Design review of the part built by this model. Coordinates are the model's own, in mm. Face numbers are marked on the shaded views. A direction names the side the tool comes from. Give positions to 0.01 mm unless a question says otherwise; leave off trailing zeros. Write each loop counter-clockwise with the first axis right and the second up, starting at its lowest first coordinate (ties: lowest second). Pieces come first, ordered by that corner, then holes.
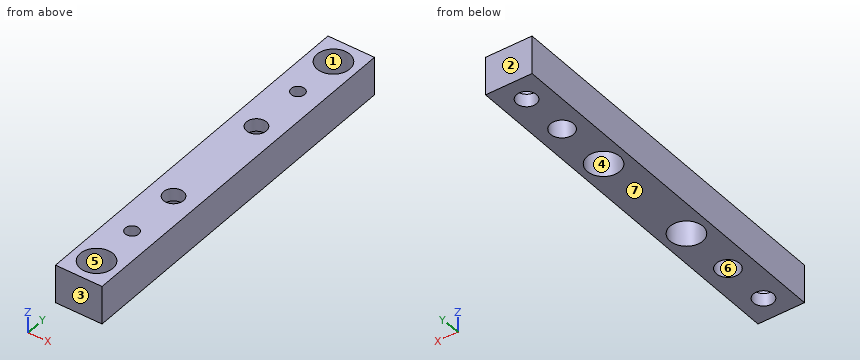
Solid Edge part; units mm, degrees
sketch "Sketch1" plane through (0, 0, 0) normal (0, 0, 1) x (1, 0, 0)
  line L0 (-7.25, -57.5) -> (7.25, -57.5)
  line L1 (7.25, -57.5) -> (7.25, 57.5)
  line L2 (7.25, 57.5) -> (-7.25, 57.5)
  line L3 (-7.25, 57.5) -> (-7.25, -57.5)
  dimension "D1" = 7.25
  dimension "D2" = 7.25
extrude "Protrusion1" add sketch "Sketch1" along normal blind 12
sketch "Sketch2" plane through (0, 0, 0) normal (0, 0, -1) x (0, -1, 0)
  circle A0 centre (-35, 0) radius 2.1
  circle A1 centre (-50, 0) radius 3.1
  circle A2 centre (-17.5, 0) radius 3.1
  dimension "D1" = 0
  dimension "D2" = 0
extrude "Cutout1" cut sketch "Sketch2" against normal up to next
sketch "Sketch3" plane through (0, 0, 0) normal (0, 0, -1) x (0, -1, 0)
  circle A0 centre (-17.5, 0) radius 5.1
  circle A1 centre (-35, 0) radius 3.6
extrude "ExtrudedCutout_2" cut sketch "Sketch3" against normal blind 8
sketch "Sketch4" plane through (0, 0, 12) normal (0, 0, 1) x (0, -1, 0)
  circle A0 centre (-50, 0) radius 5.1
extrude "ExtrudedCutout_3" cut sketch "Sketch4" against normal blind 8
mirror "Mirror1" about plane through (0, 0, 0) normal (0, 1, 0) of "Cutout1", "ExtrudedCutout_2", "ExtrudedCutout_3"
(1) To check wall thickness, follow L1, parallel to Y at x = 4, z = 10; L2, parallel to X at y = 35, z = 4; L3, parallel to Y at x = 3.75, z = 10.75. State the ranges of each line that lie inside material, in increasing order.
Resolved:
L1: y = -57.5 to -53.16, -46.84 to 46.84, 53.16 to 57.5
L2: x = -7.25 to -3.6, 3.6 to 7.25
L3: y = -57.5 to -53.46, -46.54 to 46.54, 53.46 to 57.5
(2) Consider section B-B, the plane y = -35. Give the boundary of the cut face in (x, z).
Resolved:
outline: (-7.25, 0) - (-3.6, 0) - (-3.6, 8) - (-2.1, 8) - (-2.1, 12) - (-7.25, 12) - close; (2.1, 8) - (3.6, 8) - (3.6, 0) - (7.25, 0) - (7.25, 12) - (2.1, 12) - close
(3) Mouldability with a two-part tool opening along Y and no side actions: class the marked faces 1, 2, 3 and 4 as pulls with the +Y half, pulls with the -Y half, needs draft (parallel to the pull), parting line crosses it, or undercut.
Resolved:
face 1: undercut
face 2: pulls with the +Y half
face 3: pulls with the -Y half
face 4: undercut
(4) Tool access review of the marked faces 5, 6 and 7: name each direction out of +Z, -Z, +X, -X, +Y, -Y from which nothing blocks a thin tool from reaching the whole face with its end or side.
Resolved:
face 5: +Z
face 6: -Z
face 7: -Z, +X, -X, +Y, -Y
(5) Consider section A-A, the plane z = 5.75. Give the boundary of the cut face in (x, y), then the cut area to 3 significant figures.
Resolved:
outline: (-7.25, -57.5) - (7.25, -57.5) - (7.25, 57.5) - (-7.25, 57.5) - close; hole circle Ø10.2 at (0, -50); hole circle Ø10.2 at (0, -17.5); hole circle Ø10.2 at (0, 17.5); hole circle Ø10.2 at (0, 50); hole circle Ø7.2 at (0, -35); hole circle Ø7.2 at (0, 35)
area: 1,260 mm2
(6) Clearance check with flat-ended pins moving along their axes: P1, Ø5, axis at x = -0.5, y = -15.5, coming from the -Z side; P2, Ø3.5, axis at x = 0, y = -17.5, coming from the +Z side; P3, Ø5, axis at x = 2, y = 19.5, coming from the -Z side; P4, Ø5, axis at x = -1.5, y = -49.5, coming from the +Z side. State where each tip first meets the part, or that it passes through.
Resolved:
P1: stops at z = 8
P2: passes through
P3: stops at z = 0
P4: stops at z = 4
(7) Consider section D-D, the plane y = 17.5. Give the boundary of the cut face in (x, z), then the cut area to 3 significant figures.
Resolved:
outline: (-7.25, 0) - (-5.1, 0) - (-5.1, 8) - (-3.1, 8) - (-3.1, 12) - (-7.25, 12) - close; (3.1, 8) - (5.1, 8) - (5.1, 0) - (7.25, 0) - (7.25, 12) - (3.1, 12) - close
area: 67.6 mm2
(8) Consider section C-C, the plane x = 0. Give the number of separate pieces and of enclosed holes in the cut face, then the cut area to 3 significant figures.
Resolved:
separate pieces: 7
enclosed holes: 0
area: 806 mm2
